Design review of the part built by this model. Coordinates are the model's own, in mm. Face numbers are marked on the shaded views. A direction names the side the tool comes from. Round coordinates to 2 decimals unless told otherwise and drop trailing zeros. Loops run counter-clockwise (first coordinate to the right, second up) from the corner with the lowest first, then second, coordinate; pieces in that order, holes last. Notation, with made-up numbers: (85, -15) -> (119, -15) arc R26 ccw to (119, 22) -> close; hole circle Ø11 at (25.5, 9). An arc over 180 degrees is marked (long way). Write each question's results on one line, items separated by ' | '. Start each with the question number.
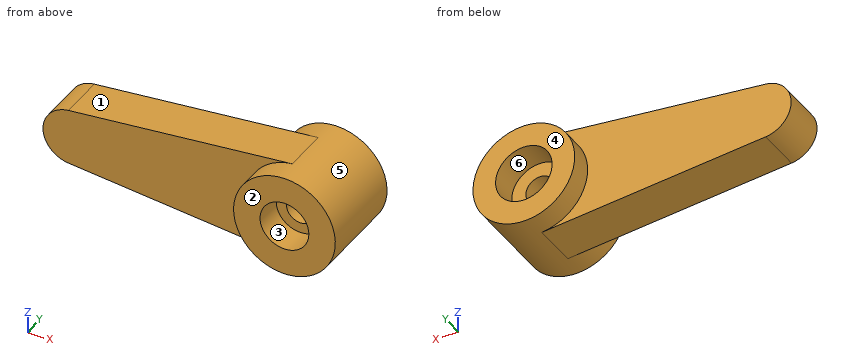
from build123d import *

# Parameters (mm, degrees)
SALIENTE_EXTRUIR1_DEPTH      = 2
SALIENTE_EXTRUIR1_DEPTH_BACK = 2


with BuildPart() as part:
    # Croquis1 → Revolución1 (revolve)
    with BuildSketch(Plane(origin=(0, 0, 0), x_dir=(0, 0, -1), z_dir=(1, 0, 0))):
        Polygon((-4.5, 4), (-4.5, -4), (-2.158881548, -4), (-2.158881548, -1.5), (-1.25, -1.5), (-1.25, 1.5), (-2.5, 1.5), (-2.5, 4), align=None)
    revolve(axis=Axis((0, 9.054619894, 0), (0, -1, 0)))

    # Croquis2 → Saliente-Extruir1 (add, two sides)
    with BuildSketch(Plane(origin=(0, 0, 0), x_dir=(1, 0, 0), z_dir=(0, 1, 0))) as saliente_extruir1_sk:
        with BuildLine():
            Line((-20.25, 2.487468593), (-0.45, 4.477443467))
            ThreePointArc((-0.45, 4.477443467), (-4.5, 0), (-0.45, -4.477443467))
            Line((-0.45, -4.477443467), (-20.25, -2.487468593))
            ThreePointArc((-20.25, -2.487468593), (-22.5, 0), (-20.25, 2.487468593))
        make_face()
    extrude(amount=SALIENTE_EXTRUIR1_DEPTH)
    extrude(saliente_extruir1_sk.sketch, amount=-SALIENTE_EXTRUIR1_DEPTH_BACK)


solid = part.part
1) Take a section at D-D (z = -4). Write out the cut boundary in (x, y).
2) The part is to be moulded in two halves that separate along X. For the marked faces 1, 2 and 3, say which applies: +X half, -X half, draft (parallel to the pull), parting line (faces both ways), or undercut.
3) Insertion check: pin 1 (2.5 mm diameter, centred on x = -1, z = 0, fed in from +Y); pin 2 (2 mm diameter, centred on x = -1, z = 0.5, fed in from -Y); pin 3 (4.5 mm diameter, centred on x = -7, z = 0, fed in from -Y). Each pin has a flat end and moves straight along its axis. Give the tip position at first contact, or say it passes through.
4) To check wall thickness, follow line 1 (X direction, y = 0.15, z = 0); line 2 (X direction, y = -2.05, z = 0); line 3 (Z direction, x = 0, y = 3.35). State the ranges of each line that lie inside material, in increasing order. Write a range as from..to.
5) Take a section at B-B (z = 0). Write out the cut boundary in (x, y).
6) Take a section at C-C (y = 0.5). Write out the cut boundary in (x, z).
7) Take a section at A-A (x = 0). Write out the cut boundary in (y, z), plus the area to 3 significant figures.
8) For the marked faces 4, 5 and 6, list the 3-axis set-ups (+Z, -Z, +X, -X, +Y, -Y) from which the entire face can be reached by the end or side of a thin tool; tool diameter is ignored.
Geometry check:
1) outline: (-5.2, -2) -> (-2.06, -2) -> (-2.06, -4) -> (2.06, -4) -> (2.06, 4) -> (-2.06, 4) -> (-2.06, 2) -> (-5.2, 2) -> close
2) face 1: -X half | face 2: draft | face 3: undercut
3) pin 1: stops at y = 1.5 | pin 2: stops at y = -1.5 | pin 3: stops at y = -2
4) line 1: x = -22.5..-1.25, 1.25..4.5 | line 2: x = -4.5..-2.16, 2.16..4.5 | line 3: z = -4.5..-2.5, 2.5..4.5
5) outline: (-22.5, -2) -> (-4.5, -2) -> (-4.5, -4) -> (-2.16, -4) -> (-2.16, -1.5) -> (-1.25, -1.5) -> (-1.25, 1.5) -> (-2.5, 1.5) -> (-2.5, 4) -> (-4.5, 4) -> (-4.5, 2) -> (-22.5, 2) -> close; (1.25, -1.5) -> (2.16, -1.5) -> (2.16, -4) -> (4.5, -4) -> (4.5, 4) -> (2.5, 4) -> (2.5, 1.5) -> (1.25, 1.5) -> close
6) outline: (-20.25, -2.49) -> (-0.45, -4.48) arc R4.5 ccw (long way) to (-0.45, 4.48) -> (-20.25, 2.49) arc R2.5 ccw to start; hole circle Ø2.5 at (0, 0)
7) outline: (-4, -4.5) -> (4, -4.5) -> (4, -2.5) -> (1.5, -2.5) -> (1.5, -1.25) -> (-1.5, -1.25) -> (-1.5, -2.16) -> (-4, -2.16) -> close; (-4, 2.16) -> (-1.5, 2.16) -> (-1.5, 1.25) -> (1.5, 1.25) -> (1.5, 2.5) -> (4, 2.5) -> (4, 4.5) -> (-4, 4.5) -> close | area: 41.2 mm^2
8) face 4: +Z, -Z, +X, -X, +Y | face 5: none | face 6: +Y
